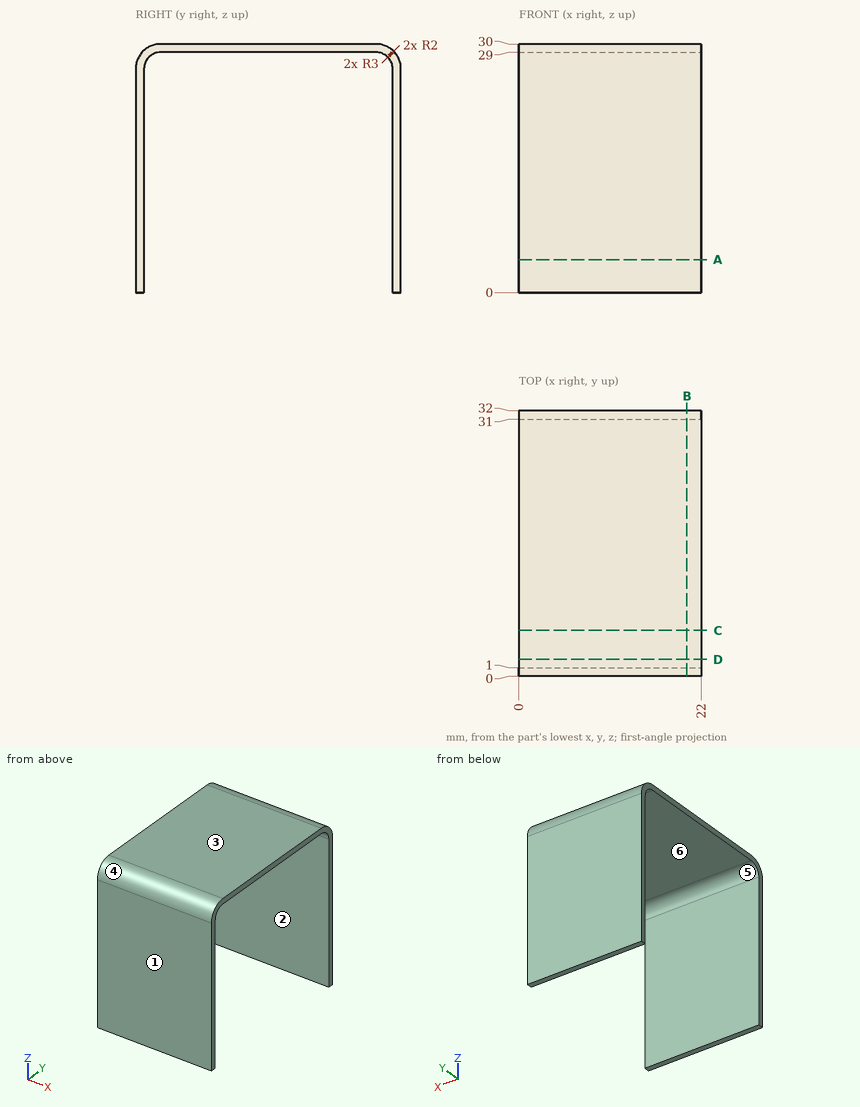
Here's the drawing with two shaded views (mm, measured from the low corner). I have some questions. A direction names the side the tool comes from. Round coordinates to 2 decimals unless told otherwise and drop trailing zeros. Order: outer loops, then holes, each group sorted by start corner. A loop starts at its lowest first (then second) coordinate and runs counter-clockwise, first axis right, second up. Notation, with made-up numbers: (-36.5, 26) -> (17.5, 26) arc R13 cw to (17.5, 37) -> close; hole circle Ø2 at (-5, 71). An arc over 180 degrees is marked (long way). Use a Markdown table: item, result. Add a question column.
(1) Suppose I cut it at D-D, the plane y = 2. Please give me the cut outline in (x, z), and give its area (3 significant figures).
(2) Suppose I cut it at A-A, the plane z = 4. Please give me the cut outline in (x, y).
(3) Suppose I cut it at C-C, the plane y = 5.5. Please give me the cut outline in (x, z).
(4) Suppose I cut it at B-B, the plane x = 20.25. Please give me the cut outline in (y, z).
(5) For the marked faces 1 and 2, which set-ups out of +Z, -Z, +X, -X, +Y, -Y let a thin tool reach every point of the face, with its end or its side?
(6) I need wall thicknesses on line 1 along Y through (x, z) = (15.25, 20); line 2 along Z through (x, y) = (12.5, 20); line 3 along Y through (x, z) = (9.5, 28). Which ranges of each line are inside material? Lowest first, please.
(7) If we mould it in two halves opening along Y, with no side actions, what happens to the marked faces 3, 4, 5 and 6? For each: released by +Y, released by -Y, zero draft, split by the parting line, or undercut.
(8) For pin 1 Ø2 at (x, z) = (6, 18.5) entering from -Y; pin 2 Ø11 at (x, y) = (9, 19) entering from -Z, each with a flat end and sliding along its axis, tell me the tip position at first contact or that it passes through.
Verdict:
| question | item | result |
|---|---|---|
| 1 | outline | (0, 28.73) -> (22, 28.73) -> (22, 29.83) -> (0, 29.83) -> close |
| 1 | area | 24.1 mm2 |
| 2 | outline | (0, 0) -> (22, 0) -> (22, 1) -> (0, 1) -> close; (0, 31) -> (22, 31) -> (22, 32) -> (0, 32) -> close |
| 3 | outline | (0, 29) -> (22, 29) -> (22, 30) -> (0, 30) -> close |
| 4 | outline | (0, 0) -> (1, 0) -> (1, 27) arc R2 cw to (3, 29) -> (29, 29) arc R2 cw to (31, 27) -> (31, 0) -> (32, 0) -> (32, 27) arc R3 ccw to (29, 30) -> (3, 30) arc R3 ccw to (0, 27) -> close |
| 5 | face 1 | +Z, -Z, +X, -X, -Y |
| 5 | face 2 | -Z, +X, -X |
| 6 | line 1 | 0 to 1, 31 to 32 |
| 6 | line 2 | 29 to 30 |
| 6 | line 3 | 0.17 to 1.27, 30.73 to 31.83 |
| 7 | face 3 | zero draft |
| 7 | face 4 | released by -Y |
| 7 | face 5 | undercut |
| 7 | face 6 | undercut |
| 8 | pin 1 | y = 0 |
| 8 | pin 2 | z = 29 |
